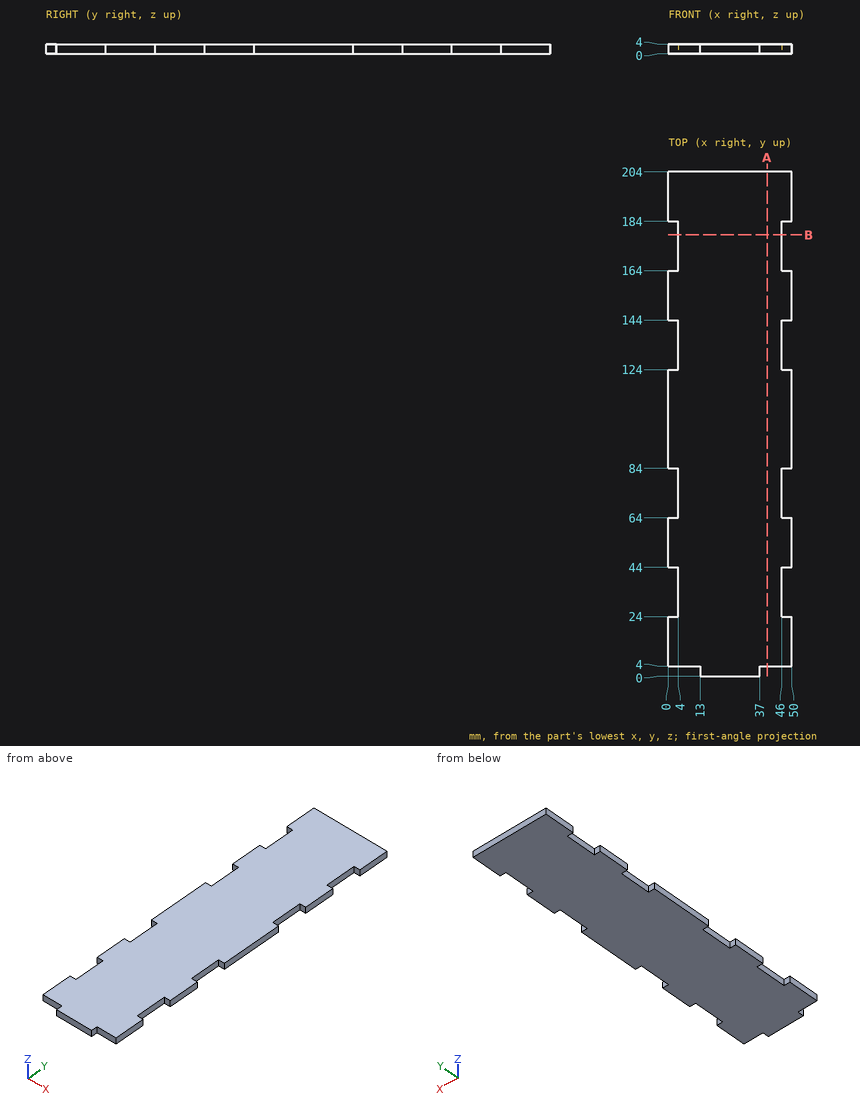
Study the drawing (mm; zero at the part's minimum x, y, z) and answer. Give positions to 0.01 mm unless a question says otherwise; leave off trailing zeros. Loops run counter-clockwise (first coordinate to the right, second up) from the corner with the lowest first, then second, coordinate; pieces in that order, holes last. Notation, with made-up numbers: (72, -36) - (86, -36) arc R13 ccw to (86, -22) - close; hole circle Ø4 at (-31.75, 6.5). An arc over 180 degrees is marked (long way). Return JSON: item names as keys, results as strings. Group by question number.
1. Find section A-A (x = 40). Write down the section's boundary in (y, z).
2. Find section B-B (y = 178.5). Write down the section's boundary in (x, z), then the cut area to 3 significant figures.
3. Straight lines are drawn through the part: line 1 (Y direction, x = 47.5, z = 2.05); line 2 (X direction, y = 30, z = 0.5); line 3 (Y direction, x = 45.5, z = 2.5). For each, find the intervals that lie inside material, in ascending order. Write a range as [from, to].
4. Given pin 1 Ø2 at (y, z) = (2, 1.5) entering from +X; pin 2 Ø1.2 at (x, z) = (47.5, 1) entering from -Y; pin 3 Ø1.2 at (y, z) = (72.5, 2) entering from -X, each flat-ended and moving along its own axis, determine where each tip first touches the part or whether it passes through.
Verdict:
{
 "1": {"outline": "(4, 0) - (204, 0) - (204, 4) - (4, 4) - close"},
 "2": {"outline": "(4, 0) - (46, 0) - (46, 4) - (4, 4) - close", "area": "168 mm^2"},
 "3": {"line 1": "y = [4, 24], [44, 64], [84, 124], [144, 164], [184, 204]", "line 2": "x = [4, 46]", "line 3": "y = [4, 204]"},
 "4": {"pin 1": "stops at x = 37", "pin 2": "stops at y = 4", "pin 3": "stops at x = 4"}
}
